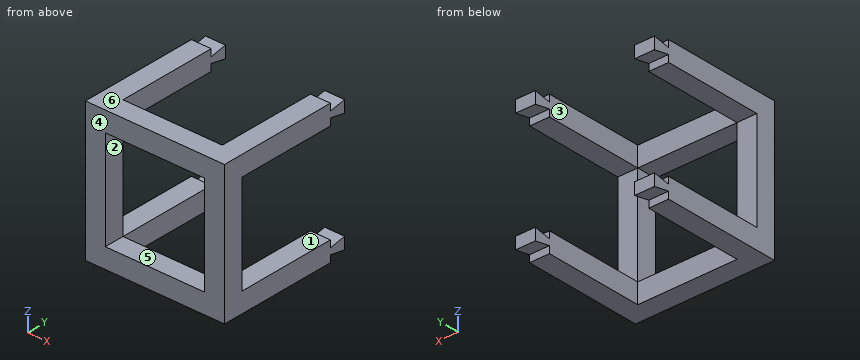
Autodesk Fusion 360 part; units mm, degrees
sketch "Sketch1" plane through (0, 0, 0) normal (0, 1, 0) x (1, 0, 0)
  line L0 (5.1128, -4.9272) -> (94.0128, -4.9272)
  line L1 (94.0128, -4.9272) -> (94.0128, -93.8272)
  line L2 (94.0128, -93.8272) -> (5.1128, -93.8272)
  line L3 (5.1128, -93.8272) -> (5.1128, -4.9272)
  line L4 (17.8128, -17.6272) -> (81.3128, -17.6272)
  line L5 (81.3128, -17.6272) -> (81.3128, -81.1272)
  line L6 (81.3128, -81.1272) -> (17.8128, -81.1272)
  line L7 (17.8128, -81.1272) -> (17.8128, -17.6272)
  dimension "d1" = 88.9
  dimension "d2" = 88.9
  dimension "d3" = 12.7
  dimension "d4" = 12.7
  dimension "d5" = 12.7
  dimension "d6" = 12.7
extrude "Extrude1" add sketch "Sketch1" along normal blind 88.9
sketch "Sketch2" plane through (0, 0, 93.8272) normal (0, 0, 1) x (1, 0, 0)
  line L0 (5.1128, 0) -> (94.0128, 0)
  line L1 (94.0128, 0) -> (94.0128, 88.9)
  line L2 (94.0128, 88.9) -> (5.1128, 88.9)
  line L3 (5.1128, 88.9) -> (5.1128, 0)
  line L4 (17.8128, 76.2) -> (81.3128, 76.2)
  line L5 (81.3128, 76.2) -> (81.3128, 12.7)
  line L6 (81.3128, 12.7) -> (17.8128, 12.7)
  line L7 (17.8128, 12.7) -> (17.8128, 76.2)
  dimension "d9" = 12.7
  dimension "d10" = 12.7
  dimension "d11" = 12.7
  dimension "d12" = 12.7
extrude "Extrude2" cut sketch "Sketch2" against normal blind 88.9 contours L4 L5 L6 L7
sketch "Sketch3" plane through (5.1128, 0, 0) normal (-1, 0, 0) x (0, 0, 1)
  line L0 (4.9272, 0) -> (93.8272, 0)
  line L1 (93.8272, 0) -> (93.8272, 88.9)
  line L2 (93.8272, 88.9) -> (4.9272, 88.9)
  line L3 (4.9272, 88.9) -> (4.9272, 0)
  line L4 (17.6272, 76.2) -> (81.1272, 76.2)
  line L5 (81.1272, 76.2) -> (81.1272, 12.7)
  line L6 (81.1272, 12.7) -> (17.6272, 12.7)
  line L7 (17.6272, 12.7) -> (17.6272, 76.2)
  dimension "d15" = 12.7
  dimension "d16" = 12.7
  dimension "d17" = 12.7
  dimension "d18" = 12.7
extrude "Extrude3" cut sketch "Sketch3" against normal blind 88.9 contours L4 L5 L6 L7
sketch "Sketch4" plane through (5.1128, 0, 0) normal (-1, 0, 0) x (0, 0, 1)
  line L0 (81.1272, 76.2) -> (81.1272, 12.7)
  line L1 (81.1272, 12.7) -> (17.6272, 12.7)
  line L2 (17.6272, 12.7) -> (17.6272, 76.2)
  line L3 (17.6272, 76.2) -> (81.1272, 76.2)
  line L4 (4.9272, 0) -> (93.8272, 0)
  line L5 (93.8272, 0) -> (93.8272, 88.9)
  line L6 (93.8272, 88.9) -> (4.9272, 88.9)
  line L7 (4.9272, 88.9) -> (4.9272, 0)
  line L8 (17.6272, 76.2) -> (81.1272, 76.2)
  line L9 (81.1272, 88.9) -> (17.6272, 88.9)
  line L10 (17.6272, 76.2) -> (4.9272, 76.2) construction
  line L11 (11.2772, 76.2) -> (11.2772, 88.9) construction
  line L12 (17.6272, 76.2) -> (13.1822, 76.2)
  line L13 (4.9272, 76.2) -> (9.3722, 76.2)
  line L14 (17.6272, 88.9) -> (15.0872, 88.9) construction
  line L15 (4.9272, 88.9) -> (7.4672, 88.9)
  line L16 (7.4672, 88.9) -> (7.4672, 86.36) construction
  line L17 (15.0872, 88.9) -> (15.0872, 86.36) construction
  line L18 (9.3722, 76.2) -> (7.4672, 86.36)
  line L19 (7.4672, 86.36) -> (15.0872, 86.36)
  line L20 (13.1822, 76.2) -> (15.0872, 86.36)
  line L21 (81.1272, 76.2) -> (93.8272, 76.2) construction
  line L22 (87.4772, 76.2) -> (87.4772, 88.9) construction
  line L23 (81.1272, 76.2) -> (85.5722, 76.2)
  line L24 (93.8272, 76.2) -> (89.3822, 76.2)
  line L25 (81.1272, 88.9) -> (83.6672, 88.9) construction
  line L26 (93.8272, 88.9) -> (91.2872, 88.9) construction
  line L27 (91.2872, 88.9) -> (91.2872, 86.36) construction
  line L28 (83.6672, 88.9) -> (83.6672, 86.36) construction
  line L29 (85.5722, 76.2) -> (83.6672, 86.36)
  line L30 (91.2872, 86.36) -> (89.3822, 76.2)
  line L31 (91.2872, 86.36) -> (83.6672, 86.36)
  dimension "d21" = 4.445
  dimension "d22" = 4.445
  dimension "d23" = 2.54
  dimension "d24" = 2.54
  dimension "d25" = 2.54
  dimension "d26" = 2.54
  dimension "d27" = 4.445
  dimension "d28" = 4.445
  dimension "d30" = 2.54
  dimension "d31" = 2.54
  dimension "d32" = 2.54
sketch "Sketch5" plane through (0, 0, 4.9272) normal (0, 0, -1) x (-1, 0, 0)
  line L0 (-81.3128, 12.7) -> (-81.3128, 76.2)
  line L1 (-81.3128, 76.2) -> (-17.8128, 76.2)
  line L2 (-17.8128, 76.2) -> (-17.8128, 12.7)
  line L3 (-17.8128, 12.7) -> (-81.3128, 12.7)
  line L4 (-94.0128, 0) -> (-5.1128, 0)
  line L5 (-5.1128, 0) -> (-5.1128, 88.9)
  line L6 (-5.1128, 88.9) -> (-94.0128, 88.9)
  line L7 (-94.0128, 88.9) -> (-94.0128, 0)
  line L8 (-81.3128, 76.2) -> (-17.8128, 76.2)
  line L9 (-17.8128, 76.2) -> (-17.8128, 88.9)
  line L10 (-17.8128, 88.9) -> (-81.3128, 88.9)
  line L11 (-81.3128, 88.9) -> (-81.3128, 76.2)
extrude "Extrude4" cut sketch "Sketch5" against normal blind 88.9 contours L1 L6 L8 L9 L10 L11
extrude "Extrude5" cut sketch "Sketch4" against normal blind 88.9 contours L3 L5 L6 L7 L8 L9 L12 L13 L15 L18 L19 L20 L23 L24 L29 L30 L31
CAD build for the part. Positions are in the model's coordinates, mm. Face numbers are marked on the shaded views. A direction names the side the tool comes from. Round coordinates to 2 decimals unless told otherwise and drop trailing zeros. Order: outer loops, then holes, each group sorted by start corner. A loop starts at its lowest first (then second) coordinate and runs counter-clockwise, first axis right, second up. Notation, with made-up numbers: (-26, 39.25) -> (-22, 39.25) arc R17 ccw to (-22, 51.25) -> close; hole circle Ø3 at (65, -9). An arc over 180 degrees is marked (long way). Write item = value, one per line.
(1) Cut at C-C (y = 10). Write the cut outline in (x, z), plus the area to 3 significant figures.
Answers follow:
outline = (5.11, 4.93) -> (94.01, 4.93) -> (94.01, 93.83) -> (5.11, 93.83) -> close; hole (17.81, 17.63) -> (81.31, 17.63) -> (81.31, 81.13) -> (17.81, 81.13) -> close
area = 3,870 mm²
(2) Cut at A-A (x = 73). Write the cut outline in (y, z).
Answers follow:
outline = (0, 4.93) -> (12.7, 4.93) -> (12.7, 17.63) -> (0, 17.63) -> close; (0, 81.13) -> (12.7, 81.13) -> (12.7, 93.83) -> (0, 93.83) -> close
(3) Cut at D-D (y = 39). Write the cut outline in (x, z).
Answers follow:
outline = (5.11, 4.93) -> (17.81, 4.93) -> (17.81, 17.63) -> (5.11, 17.63) -> close; (5.11, 81.13) -> (17.81, 81.13) -> (17.81, 93.83) -> (5.11, 93.83) -> close; (81.31, 4.93) -> (94.01, 4.93) -> (94.01, 17.63) -> (81.31, 17.63) -> close; (81.31, 81.13) -> (94.01, 81.13) -> (94.01, 93.83) -> (81.31, 93.83) -> close
(4) Cut at B-B (z = 68.5). Write the cut outline in (x, y).
Answers follow:
outline = (5.11, 0) -> (17.81, 0) -> (17.81, 12.7) -> (5.11, 12.7) -> close; (81.31, 0) -> (94.01, 0) -> (94.01, 12.7) -> (81.31, 12.7) -> close
(5) Drill centre lines: L1, parallel to Z at x = 83.5, y = 62.5; L2, parallel to X at y = 19, z = 15.5; L3, parallel to Y at x = 71, z = 11. Where is each one in solid material? Low to high.
Answers follow:
L1 = 4.93 to 17.63, 81.13 to 93.83
L2 = 5.11 to 17.81, 81.31 to 94.01
L3 = 0 to 12.7
(6) 3-axis set-ups, long thin cutter, end or side, ignore diameter. For the marked faces 1, 2 and 3: which of +Z, -Z, +X, -X, +Y, -Y reach the whole face in a straight line?
Answers follow:
face_1 = +X, -X, +Y
face_2 = +Y, -Y
face_3 = +Z, -Z, +Y
(7) Pull direction Z, two halves, no side cores. Call the marked faces 4, 5 and 6: +Z half, -Z half, draft (parallel to the pull), parting line (faces both ways), or undercut.
Answers follow:
face_4 = draft
face_5 = undercut
face_6 = +Z half
(8) Flat gauge pin, fed straight in: P1, Ø10, axis at x = 43, z = 11, coming from the +Y side. Where does the tip first touch, or does it go through?
Answers follow:
P1 = 12.7
